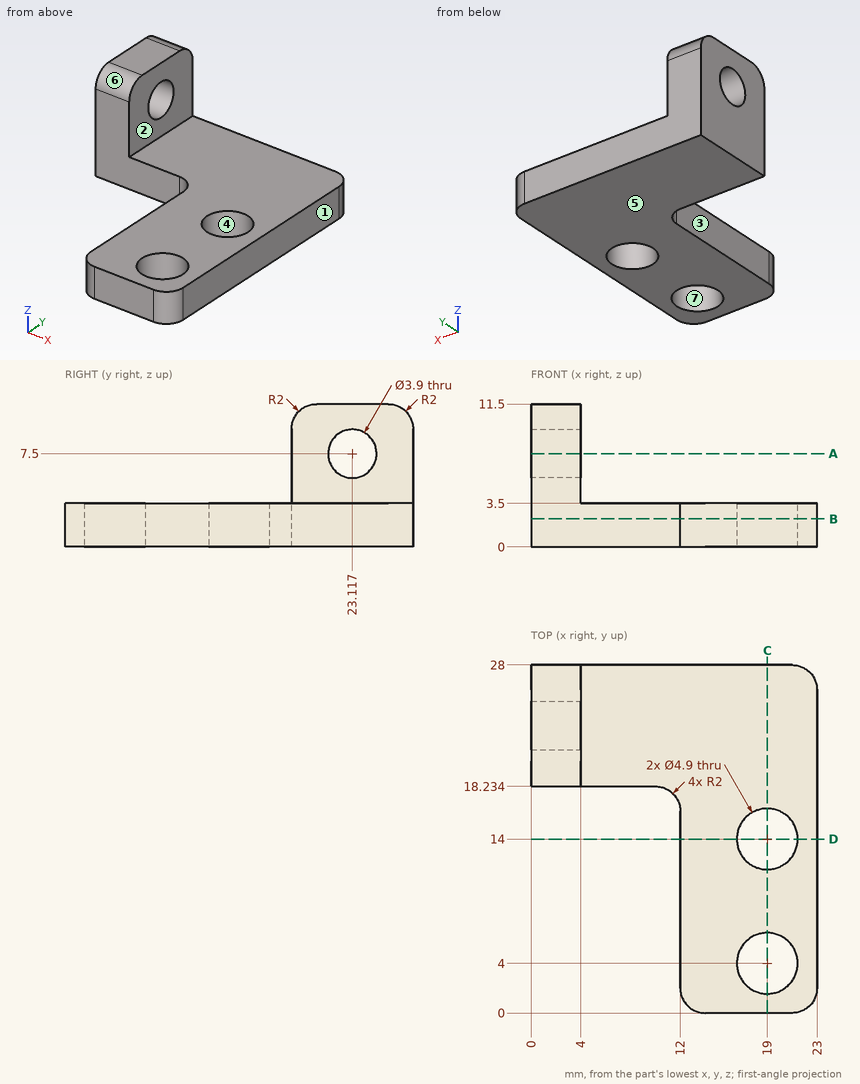
Geometry: see drawing. Coordinates: mm, zero at the bounding-box minimum. A direction names the side the tool comes from. Coordinates: 2 decimals unless noted, no trailing zeros. Order: outer loops, then holes, each group sorted by start corner. A loop starts at its lowest first (then second) coordinate and runs counter-clockwise, first axis right, second up. Notation, with made-up numbers: (80, 84.5) -> (120, 84.5) arc R19 ccw to (120, 96.5) -> close; hole circle Ø6 at (-7, 17). An arc over 180 degrees is marked (long way). Write each question's results on one line, items separated by ' | '. Start each with the question number.
1) First-contact query: pin 1 (1.5 mm diameter, centred on x = 11.5, z = 4, fed in from +Y); pin 2 (4.5 mm diameter, centred on y = 23.12, z = 7.5, fed in from +X); pin 3 (3 mm diameter, centred on y = 8.5, z = 1.5, fed in from -X); pin 4 (2 mm diameter, centred on x = 17, y = 20.5, fed in from +Z). Flat tips, straight axial feed; report the tip coordinate or a pass-through.
2) Cut plane A-A, the plane z = 7.5. Output: boundary loops of the cut face in (x, y).
3) Cut plane C-C, the plane x = 19. Output: boundary loops of the cut face in (y, z).
4) Set-up query: the marked faces 1, 2 and 3. Return all of +Z, -Z, +X, -X, +Y, -Y with unobstructed straight access to the full face (end or side cutting, diameter ignored); none if empty.
5) Material intervals for line 1 along Y through (x, z) = (19, 1.35); line 2 along Y through (x, z) = (3.1, 7.5); line 3 along Z through (x, y) = (9, 20.5), sorted ascending.
6) Cut plane D-D, the plane y = 14. Output: boundary loops of the cut face in (x, z).
7) Cut plane B-B, the plane z = 2.25. Output: boundary loops of the cut face in (x, y).
8) Mould query, pull axis Y, two halves, no side actions, for the marked faces 4, 5, 6 and 7. Classes: released by +Y, released by -Y, zero draft, split by the parting line, or undercut.
Checks:
1) pin 1: y = 28 | pin 2: x = 4 | pin 3: x = 12 | pin 4: z = 3.5
2) outline: (0, 18.23) -> (4, 18.23) -> (4, 21.17) -> (0, 21.17) -> close; (0, 25.07) -> (4, 25.07) -> (4, 28) -> (0, 28) -> close
3) outline: (0, 0) -> (1.55, 0) -> (1.55, 3.5) -> (0, 3.5) -> close; (6.45, 0) -> (11.55, 0) -> (11.55, 3.5) -> (6.45, 3.5) -> close; (16.45, 0) -> (28, 0) -> (28, 3.5) -> (16.45, 3.5) -> close
4) face 1: +Z, -Z, +X, +Y, -Y | face 2: +Z, +X, +Y, -Y | face 3: +Z, -Z, -X, -Y
5) line 1: 0 to 1.55, 6.45 to 11.55, 16.45 to 28 | line 2: 18.23 to 21.17, 25.07 to 28 | line 3: 0 to 3.5
6) outline: (12, 0) -> (16.55, 0) -> (16.55, 3.5) -> (12, 3.5) -> close; (21.45, 0) -> (23, 0) -> (23, 3.5) -> (21.45, 3.5) -> close
7) outline: (0, 18.23) -> (10, 18.23) arc R2 cw to (12, 16.23) -> (12, 2) arc R2 ccw to (14, 0) -> (21, 0) arc R2 ccw to (23, 2) -> (23, 26) arc R2 ccw to (21, 28) -> (0, 28) -> close; hole circle Ø4.9 at (19, 4); hole circle Ø4.9 at (19, 14)
8) face 4: undercut | face 5: zero draft | face 6: released by -Y | face 7: undercut
